Here's how the part is built. I have some questions about the finished solid (model axes, mm). A direction names the side the tool comes from. Round coordinates to 2 decimals unless told otherwise and drop trailing zeros. Loops run counter-clockwise (first coordinate to the right, second up) from the corner with the lowest first, then second, coordinate; pieces in that order, holes last. Notation, with made-up numbers: M -13,46 L 7,46 A23 ccw 7,73 Z; hole C -7.75,-24 d2. An arc over 180 degrees is marked long. Answer as a JSON object with one key per item and string values.
Autodesk Inventor part; units mm, degrees
ref_plane "YZ Plane" through (0, 0, 0) normal (1, 0, 0) x (0, 1, 0)
ref_plane "XZ Plane" through (0, 0, 0) normal (0, 1, 0) x (-1, 0, 0)
ref_plane "XY Plane" through (0, 0, 0) normal (0, 0, 1) x (1, 0, 0)
sketch "Sketch1" plane through (0, 0, 0) normal (0, 1, 0) x (-1, 0, 0)
  line L0 (-45.5, -29.5) -> (45.5, -29.5)
  line L1 (45.5, -29.5) -> (45.5, 29.5)
  line L2 (45.5, 29.5) -> (-45.5, 29.5)
  line L3 (-45.5, 29.5) -> (-45.5, -29.5)
  line L4 (-45.5, -29.5) -> (45.5, 29.5) construction
  line L5 (45.5, -29.5) -> (-45.5, 29.5) construction
  point P0 (0, 0)
  dimension "d0" = 91
  dimension "d1" = 59
extrude "Extrusion1" add sketch "Sketch1" along normal blind 3
sketch "Sketch2" plane through (0, 3, 0) normal (0, 1, 0) x (1, 0, 0)
  line L0 (45.5, 29.5) -> (-45.5, 29.5)
  line L1 (-45.5, 29.5) -> (-43, 29.5)
  line L2 (-43, 29.5) -> (-43, 22.5)
  line L3 (-43, 22.5) -> (-45.5, 22.5)
  line L4 (-45.5, 22.5) -> (-45.5, 29.5)
  line L5 (-43, 22.5) -> (5, 22.5)
  line L6 (5, 22.5) -> (5, 2.1)
  line L7 (5, 2.1) -> (-43, 2.1)
  line L8 (-43, 2.1) -> (-43, 22.5)
  line L9 (6.7, 19.2) -> (28.8, 19.2)
  line L10 (28.8, 19.2) -> (28.8, 3.9)
  line L11 (28.8, 3.9) -> (6.7, 3.9)
  line L12 (6.7, 3.9) -> (6.7, 19.2)
  line L13 (6.7, 19.2) -> (28.8, 3.9) construction
  line L14 (28.8, 19.2) -> (6.7, 3.9) construction
  line L15 (3.7, -4.4) -> (33, -4.4)
  line L16 (33, -4.4) -> (33, -16.8)
  line L17 (33, -16.8) -> (3.7, -16.8)
  line L18 (3.7, -16.8) -> (3.7, -4.4)
  line L19 (3.7, -4.4) -> (33, -16.8) construction
  line L20 (33, -4.4) -> (3.7, -16.8) construction
  line L21 (45.5, -29.5) -> (45.5, 29.5)
  line L22 (-45.5, -29.5) -> (45.5, -29.5)
  point P0 (0, 0)
  point P1 (17.75, 11.55)
  point P2 (18.35, -10.6)
  dimension "d4" = 2.5
  dimension "d5" = 7
  dimension "d6" = 48
  dimension "d7" = 20.4
  dimension "d10" = 1.7
  dimension "d11" = 22.1
  dimension "d12" = 15.3
  dimension "d13" = 3.3
  dimension "d14" = 12.4
  dimension "d15" = 29.3
  dimension "d16" = 12.5
  dimension "d17" = 12.7
extrude "Extrusion2" add sketch "Sketch2" along normal blind 10 contours L5 L6 L7 L8 | L9 L10 L11 L12 | L15 L16 L17 L18
sketch "Sketch3" plane through (0, 3, 0) normal (0, 1, 0) x (1, 0, 0)
  line L0 (-42.5, 26.5) -> (42.5, 26.5)
  line L1 (42.5, 26.5) -> (42.5, -26.5)
  line L2 (42.5, -26.5) -> (-42.5, -26.5)
  line L3 (-42.5, -26.5) -> (-42.5, 26.5)
  line L4 (-42.5, 26.5) -> (42.5, -26.5) construction
  line L5 (42.5, 26.5) -> (-42.5, -26.5) construction
  circle A0 centre (42.5, -26.5) radius 1.6
  circle A1 centre (-42.5, -26.5) radius 1.6
  circle A2 centre (-42.5, 26.5) radius 1.6
  circle A3 centre (42.5, 26.5) radius 1.6
  point P0 (0, 0)
  dimension "d18" = 85
  dimension "d19" = 53
  dimension "d20" = 3.2
  dimension "d21" = 3.2
  dimension "d22" = 3.2
  dimension "d23" = 3.2
extrude "Extrusion3" cut sketch "Sketch3" against normal blind 3 contours L3 A2 L0 | L0 A2 L3 | A3 L1 L0 | L0 L1 A3 | A1 L2 L3 | L3 L2 A1 | A0 L2 L1 | L1 L2 A0
sketch "Sketch4" plane through (0, 13, 0) normal (0, 1, 0) x (1, 0, 0)
  line L0 (3.7, -4.4) -> (3.7, -16.8)
  line L1 (3.7, -4.4) -> (33, -4.4)
  line L2 (3.7, -16.8) -> (33, -16.8)
  line L3 (33, -16.8) -> (33, -4.4)
  line L4 (33, -4.4) -> (3.7, -4.4)
  line L5 (3.7, -4.4) -> (3.7, -16.8)
  point P0 (0, 0)
extrude "Extrusion4" add sketch "Sketch4" along normal blind 25
properties part number "PCB"
Item 1: I want a section at B-B, the plane x = 42.5. Please give me the cut outline in (y, z).
Resolved:
{"outline": "M 0,-29.5 L 3,-29.5 L 3,-28.1 L 0,-28.1 Z; M 0,-24.9 L 3,-24.9 L 3,24.9 L 0,24.9 Z; M 0,28.1 L 3,28.1 L 3,29.5 L 0,29.5 Z"}
Item 2: I want a section at C-C, the plane z = -17.5. Please give me the cut outline in (x, y), then the cut area to 3 significant figures.
Resolved:
{"outline": "M -45.5,0 L 45.5,0 L 45.5,3 L 28.8,3 L 28.8,13 L 6.7,13 L 6.7,3 L 5,3 L 5,13 L -43,13 L -43,3 L -45.5,3 Z", "area": "974 mm²"}
Item 3: Please list where these lines run through material, in increasing order: probe 1 along X at (y, z) = (0.6, 26.5); probe 2 along Z at (x, y) = (42.5, 2.3); probe 3 along X at (y, z) = (12.5, -8.5). Write a range as from..to.
Resolved:
{"probe 1": "-45.5..-44.1, -40.9..40.9, 44.1..45.5", "probe 2": "-29.5..-28.1, -24.9..24.9, 28.1..29.5", "probe 3": "-43..5, 6.7..28.8"}
Item 4: On a 3-axis mill with a long thin cutter (end or side, diameter ignored), from which of +Z, -Z, +X, -X, +Y, -Y can I reach the whole of each face in a straight line? I mean faces 1 (the face through (18, 20, 4.4)), 2 (the face through (-43, 8, -12)), 3 (the face through (6.7, 8, -11)), 4 (the face through (18, 13, -12)), 5 (the face through (33, 20, 11)). Say none if no direction works.
Resolved:
{"face 1": "+X, -X, +Y", "face 2": "+Z, -Z, -X, +Y", "face 3": "-Z, +Y", "face 4": "-Z, +X, -X, +Y", "face 5": "+Z, -Z, +X, +Y"}
Item 5: I want a section at A-A, the plane z = 26.5. Please give me the cut outline in (x, y).
Resolved:
{"outline": "M -45.5,0 L -44.1,0 L -44.1,3 L -45.5,3 Z; M -40.9,0 L 40.9,0 L 40.9,3 L -40.9,3 Z; M 44.1,0 L 45.5,0 L 45.5,3 L 44.1,3 Z"}
Item 6: If we mould it in two halves opening along Z, with no side actions, what happens to faces 6 (the face through (42.292, 1.521, -28.086)), 7 (the face through (1, 1, -29.5)), 8 (the face through (42.292, 1.521, 24.914)), 9 (the face through (18, 38, 11))? For each: pulls with the +Z half, pulls with the -Z half, needs draft (parallel to the pull), parting line crosses it, or undercut.
Resolved:
{"face 6": "undercut", "face 7": "pulls with the -Z half", "face 8": "undercut", "face 9": "needs draft"}
Item 7: I'm going to push flat-ended pins straight in: pin 1 Ø5 at (y, z) = (6.5, -21) entering from +X; pin 2 Ø3 at (x, z) = (-42.5, 26.5) entering from +Y; pin 3 Ø3 at (y, z) = (5.5, -8) entering from -X; pin 4 Ø1.5 at (y, z) = (7.5, 10.5) entering from +X. Where does each tip first touch, or does it pass through?
Resolved:
{"pin 1": "x = 28.8", "pin 2": "through", "pin 3": "x = -43", "pin 4": "x = 33"}
Item 8: I want a section at D-D, the plane x = -17. Please give me the cut outline in (y, z).
Resolved:
{"outline": "M 0,-29.5 L 3,-29.5 L 3,-22.5 L 13,-22.5 L 13,-2.1 L 3,-2.1 L 3,29.5 L 0,29.5 Z"}
